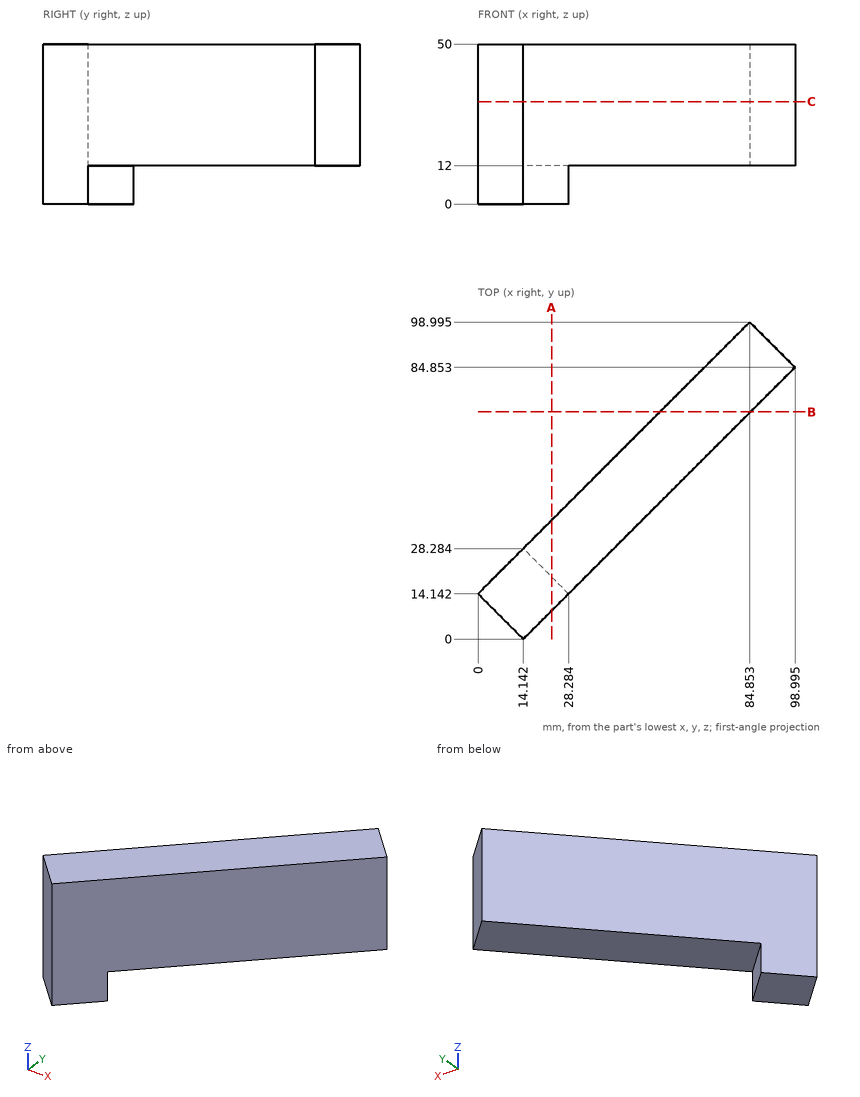
Design review of the part shown in the three views and the two pictorial views. Dimensions are in mm from the part's minimum x, y and z. Give positions to 0.01 mm unless a question says otherwise; leave off trailing zeros. Write each loop counter-clockwise with the first axis right and the second up, starting at its lowest first coordinate (ties: lowest second). Pieces come first, ordered by that corner, then holes.
Item 1: Take a section at B-B (y = 71). Give the boundary of the cut face in (x, z), and give its area (3 significant figures).
Item 2: Take a section at C-C (z = 32). Give the boundary of the cut face in (x, y) (1 decimal).
Item 3: Take a section at A-A (x = 23). Give the boundary of the cut face in (y, z).
Item 4: Insertion check: P1, Ø2, axis at x = 10.5, z = 37, coming from the +Y side; P2, Ø8, axis at x = 47, z = 18.5, coming from the -Y side; P3, Ø5, axis at x = 71.5, z = 19, coming from the -Y side. Each pin has a flat end and moves straight along its axis. Give the tip position at first contact, or say it passes through.
Item 5: Wall thickness on probe 1 along Z at (x, y) = (25, 33); probe 2 along X at (y, z) = (84.5, 43.5); probe 3 along Y at (x, z) = (9.5, 14): over which ranges is each line inside the solid? List them lowest first.
Established:
1. outline: (56.86, 12) - (85.14, 12) - (85.14, 50) - (56.86, 50) - close
1. area: 1,070 mm2
2. outline: (0, 14.1) - (14.1, 0) - (99, 84.9) - (84.9, 99) - close
3. outline: (8.86, 0) - (19.43, 0) - (19.43, 12) - (37.14, 12) - (37.14, 50) - (8.86, 50) - close
4. P1: stops at y = 25.64
4. P2: stops at y = 28.86
4. P3: stops at y = 54.86
5. probe 1: z = 12 to 50
5. probe 2: x = 70.36 to 98.64
5. probe 3: y = 4.64 to 23.64
